Input: part model. Units: mm. Frame: model coordinates. A direction names the side the tool comes from. Round coordinates to 2 decimals unless told otherwise and drop trailing zeros. Loops run counter-clockwise (first coordinate to the right, second up) from the corner with the lowest first, then second, coordinate; pieces in that order, holes last. Notation, with made-up numbers: (47.5, 84.25) - (103.5, 84.25) arc R35 ccw to (103.5, 120.25) - close; hole circle Ø8 at (14.5, 66). An arc over 180 degrees is marked (long way). One line per question, with ' | ' between items. Start each with the question number.
from build123d import *

# Parameters (mm, degrees)
F0_R     = 32.385
F0_R_2   = 28.575
F1_DEPTH = 19.05
F2_R     = 3.81
F3_DEPTH = 38.1
F6_R     = 4.445
F6_R_2   = 3.81
F7_DEPTH = 25.4
F8_R     = 4.445
F8_R_2   = 3.81
F9_DEPTH = 25.4


with BuildPart() as f1:
    # F0 (on Front) → F1 (new body)
    with BuildSketch(Plane.XZ):
        Circle(F0_R)
        Circle(F0_R_2, mode=Mode.SUBTRACT)
    extrude(amount=F1_DEPTH)

    # F2 (on Top) → F3 (cut, symmetric)
    with BuildSketch(Plane.XY):
        with Locations((0, -9.525)):
            Circle(F2_R)
    extrude(amount=F3_DEPTH, both=True, mode=Mode.SUBTRACT)

    # F6 (on offset) → F7 (cut)
    with BuildSketch(Plane.XY.offset(31.75)):
        with Locations((0, -9.525)):
            Circle(F6_R)
        with Locations((0, -9.525)):
            Circle(F6_R_2, mode=Mode.SUBTRACT)
    extrude(amount=F7_DEPTH, mode=Mode.SUBTRACT)

    # F8 (on offset) → F9 (cut)
    with BuildSketch(Plane.XY.offset(-31.75)):
        with Locations((0, -9.525)):
            Circle(F8_R)
        with Locations((0, -9.525)):
            Circle(F8_R_2, mode=Mode.SUBTRACT)
    extrude(amount=-F9_DEPTH, mode=Mode.SUBTRACT)


solid = f1.part
(1) Line query: line 1 along X through (y, z) = (-6.5, 0.5); line 2 along Y through (x, z) = (0, 30.6) (3 decimals); line 3 along X through (y, z) = (-15.25, -2). Output: solid intervals per line, ascending. Write a range as from..to.
(2) Section A-A, the plane z = 0. Output: boundary loops of the cut face in (x, y) (3 decimals), plus the area to 3 significant figures.
(3) Pull-direction query (Z, two-part tool) for faces 1 (the face through (4, -8, 31.75)), 2 (the face through (4, -8, -31.75)), 3 (the face through (-6.194, -9.392, -27.895)); classes: released by +Z, released by -Z, zero draft, split by the parting line, or undercut.
(4) Reachability of faces 4 (the face through (-3.276, -6.521, 31.996)), 5 (the face through (-7.02, -9.392, -31.615)), 6 (the face through (-3.276, -6.521, -31.996)) from +Z, -Z, +X, -X, +Y, -Y: full face, straight path, thin tool, end or side. Return the list, or none.
(5) Section B-B, the plane x = 0. Output: boundary loops of the cut face in (y, z) (3 decimals), plus the area to 3 significant figures.
(6) Section C-C, the plane y = -11. Output: boundary loops of the cut face in (x, z) (3 decimals).
(7) Pin query (flat end, axial travel): P1, Ø10, axis at x = 0, y = -9.525, coming from the +Z side (3 decimals); P2, Ø1, axis at y = -14.5, z = -4.5, coming from the -X side; P3, Ø3, axis at y = -7.5, z = 25.5, coming from the +X side; P4, Ø10, axis at x = -20.5, y = -8.5, coming from the -Z side. Return the tip coordinate at first contact, or that it passes through.
(8) Section D-D, the plane x = 26.5. Output: boundary loops of the cut face in (y, z).
Derived:
1) line 1: x = -32.38..-28.57, 28.57..32.38 | line 2: y = -19.05..-13.335, -5.715..0 | line 3: x = -32.32..-28.5, 28.5..32.32
2) outline: (-32.385, -19.05) - (-28.575, -19.05) - (-28.575, 0) - (-32.385, 0) - close; (28.575, -19.05) - (32.385, -19.05) - (32.385, 0) - (28.575, 0) - close | area: 145 mm²
3) face 1: released by +Z | face 2: released by -Z | face 3: undercut
4) face 4: +Z | face 5: +Y, -Y | face 6: -Z
5) outline: (-19.05, -32.385) - (-13.97, -32.385) - (-13.97, -31.75) - (-13.335, -31.75) - (-13.335, -28.575) - (-19.05, -28.575) - close; (-19.05, 28.575) - (-13.335, 28.575) - (-13.335, 31.75) - (-13.97, 31.75) - (-13.97, 32.385) - (-19.05, 32.385) - close; (-5.715, -31.75) - (-5.08, -31.75) - (-5.08, -32.385) - (0, -32.385) - (0, -28.575) - (-5.715, -28.575) - close; (-5.715, 28.575) - (0, 28.575) - (0, 32.385) - (-5.08, 32.385) - (-5.08, 31.75) - (-5.715, 31.75) - close | area: 85.5 mm²
6) outline: (-4.193, -32.112) - (-4.193, -31.75) - (-3.513, -31.75) - (-3.513, -28.358) arc R28.575 cw to (-3.513, 28.358) - (-3.513, 31.75) - (-4.193, 31.75) - (-4.193, 32.112) arc R32.385 ccw to start; (3.513, -31.75) - (4.193, -31.75) - (4.193, -32.112) arc R32.385 ccw to (4.193, 32.112) - (4.193, 31.75) - (3.513, 31.75) - (3.513, 28.358) arc R28.575 cw to (3.513, -28.358) - close
7) P1: stops at z = 32.385 | P2: stops at x = -32.14 | P3: stops at x = 21.74 | P4: stops at z = -28.43
8) outline: (-19.05, -18.62) - (0, -18.62) - (0, -10.69) - (-19.05, -10.69) - close; (-19.05, 10.69) - (0, 10.69) - (0, 18.62) - (-19.05, 18.62) - close
